from build123d import *

# Parameters (mm, degrees)
SKETCH1_R           = 3
BOSS_EXTRUDE2_DEPTH = 12.5
CUT_EXTRUDE1_DEPTH  = 2
SKETCH4_R           = 1.5
CUT_EXTRUDE4_DEPTH  = 2.5
SKETCH5_W           = 2.5
SKETCH5_H           = 4.5
BOSS_EXTRUDE3_DEPTH = 25
SKETCH6_R           = 1.500002847
CUT_EXTRUDE5_DEPTH  = 2.5
SKETCH7_R           = 1.1
CUT_EXTRUDE6_DEPTH  = 2


with BuildPart() as part:
    # Sketch1 → Boss-Extrude2 (new, symmetric)
    with BuildSketch(Plane.XY):
        Circle(SKETCH1_R)
        with BuildLine():
            Line((0, -3), (0, -0.5))
            Line((0, -0.5), (-17, -0.5))
            ThreePointArc((-17, -0.5), (-17.707106781, -0.792893219), (-18, -1.5))
            Line((-18, -1.5), (-18, -2))
            ThreePointArc((-18, -2), (-17.707106781, -2.707106781), (-17, -3))
            Line((-17, -3), (0, -3))
        make_face()
        Polygon((6.675258535, 32.098501889), (0.984807753, -0.173648178), (-0.984807753, 0.173648178), (4.705643029, 32.445798244), align=None)
    extrude(amount=BOSS_EXTRUDE2_DEPTH, both=True)

    # Sketch2 → Cut-Extrude1 (cut)
    with BuildSketch(Plane(origin=(0.9848077530122124, -0.17364817766692678, 0), x_dir=(0, 0, -1), z_dir=(0.9848077530122088, -0.17364817766692617, 0))):
        with BuildLine():
            Line((-8.6, 4.328427125), (8.6, 4.328427125))
            ThreePointArc((8.6, 4.328427125), (8.882842712, 4.445584412), (9, 4.728427125))
            Line((9, 4.728427125), (9, 4.928427125))
            ThreePointArc((9, 4.928427125), (8.882842712, 5.211269837), (8.6, 5.328427125))
            Line((8.6, 5.328427125), (-8.6, 5.328427125))
            ThreePointArc((-8.6, 5.328427125), (-8.882842712, 5.211269837), (-9, 4.928427125))
            Line((-9, 4.928427125), (-9, 4.728427125))
            ThreePointArc((-9, 4.728427125), (-8.882842712, 4.445584412), (-8.6, 4.328427125))
        make_face()
    extrude(amount=-CUT_EXTRUDE1_DEPTH, mode=Mode.SUBTRACT)

    # Sketch4 → Cut-Extrude4 (cut)
    with BuildSketch(Plane.XZ.offset(3)):
        with Locations((-6.562669804, 6.5)):
            Circle(SKETCH4_R)
        with Locations((-6.562669804, -6.5)):
            Circle(SKETCH4_R)
    extrude(amount=-CUT_EXTRUDE4_DEPTH, mode=Mode.SUBTRACT)

    # Sketch5 → Boss-Extrude3 (add)
    with BuildSketch(Plane.XY.offset(12.5)):
        with Locations((-1.25, -5.25)):
            Rectangle(SKETCH5_W, SKETCH5_H)
    extrude(amount=-BOSS_EXTRUDE3_DEPTH)

    # Sketch6 → Cut-Extrude5 (cut)
    with BuildSketch(Plane(origin=(0, 0, 0), x_dir=(0, 0, -1), z_dir=(1, 0, 0))):
        with Locations(Location((-8.822806399, -5.193294881, 0), (0, 0, 90))):
            Circle(SKETCH6_R)
    extrude(amount=-CUT_EXTRUDE5_DEPTH, mode=Mode.SUBTRACT)

    # Sketch7 → Cut-Extrude6 (cut)
    with BuildSketch(Plane(origin=(0.9848077530122124, -0.17364817766692678, 0), x_dir=(0, 0, -1), z_dir=(0.9848077530122088, -0.17364817766692617, 0))):
        with Locations(Location((-10.25, 30.52, 0), (0, 0, 90))):
            Circle(SKETCH7_R)
        with Locations(Location((-10.25, 17.02, 0), (0, 0, 90))):
            Circle(SKETCH7_R)
        with Locations(Location((10.25, 17.02, 0), (0, 0, 90))):
            Circle(SKETCH7_R)
        with Locations(Location((10.25, 30.52, 0), (0, 0, 90))):
            Circle(SKETCH7_R)
    extrude(amount=-CUT_EXTRUDE6_DEPTH, mode=Mode.SUBTRACT)


solid = part.part
Verification items for the finished model (mm, model axes). A direction names the side the tool comes from. Round coordinates to 2 decimals unless told otherwise and drop trailing zeros. Order: outer loops, then holes, each group sorted by start corner. A loop starts at its lowest first (then second) coordinate and runs counter-clockwise, first axis right, second up.
1. Section check B-B on z = -6.5. Record the cut outline in (x, y), then the cut area to 3 significant figures.
Final values:
outline: (-18, -2) arc R1 ccw to (-17, -3) - (-8.06, -3) - (-8.06, -0.5) - (-17, -0.5) arc R1 ccw to (-18, -1.5) - close; (-5.06, -3) - (-2.5, -3) - (-2.5, -7.5) - (0, -7.5) - (0, -3) arc R3 ccw to (1.48, 2.61) - (1.74, 4.09) - (-0.23, 4.44) - (-0.49, 2.96) arc R3 ccw to (-2.96, -0.5) - (-5.06, -0.5) - close; (-0.06, 5.42) - (1.91, 5.07) - (6.68, 32.1) - (4.71, 32.45) - close
area: 129 mm2
2. Thickness scan on L1, parallel to Y at x = -10.75, z = -9.5; L2, parallel to X at y = -5, z = -7; L3, parallel to X at y = 28, z = 6.5. Record the ranges inside material, lowest first.
Final values:
L1: y = -3 to -0.5
L2: x = -2.5 to 0
L3: x = 3.92 to 5.95
3. Section check D-D on x = -1. Record the cut outline in (y, z), then the cut area to 3 significant figures.
Final values:
outline: (-7.5, -12.5) - (2.83, -12.5) - (2.83, 12.5) - (-7.5, 12.5) - close; hole circle Ø3 at (-5.19, 8.82)
area: 251 mm2
4. Access from +Z, -Z, +X, -X, +Y, -Y to the whole of each face (thin tool, end or side, straight path). Record for faces 1 (the flat face through (-10, -3, 0)), 2 (the cylindrical face through (2.887, -0.816, 0.175)), 3 (the flat face through (0, -5, 0)), 4 (the flat face through (0.939, 5.245, -0.12)), 5 (the cylindrical face through (-1.23, -4.39, 10.09)).
Final values:
face 1: +Z, -Z, -X, -Y
face 2: +Z, -Z, +X
face 3: +Z, -Z, +X, -Y
face 4: -X
face 5: +X, -X
5. Go/stop test with flat-tipped pins: P1, Ø2, axis at x = 2.5, y = 26.5, coming from the +Z side; P2, Ø4, axis at y = 10, z = -4, coming from the -X side; P3, Ø4.5, axis at x = -11, z = 3, coming from the -Y side; P4, Ø6, axis at x = -8.5, z = -9, coming from the +Y side. Record where each tip stops, or that it passes through.
Final values:
P1: passes through
P2: stops at x = 0.4
P3: stops at y = -3
P4: stops at y = -0.5
6. Section check A-A on z = 1. Record the cut outline in (x, y).
Final values:
outline: (-18, -2) arc R1 ccw to (-17, -3) - (-2.5, -3) - (-2.5, -7.5) - (0, -7.5) - (0, -3) arc R3 ccw to (1.48, 2.61) - (1.74, 4.09) - (-0.23, 4.44) - (-0.49, 2.96) arc R3 ccw to (-2.96, -0.5) - (-17, -0.5) arc R1 ccw to (-18, -1.5) - close; (-0.06, 5.42) - (1.91, 5.07) - (6.68, 32.1) - (4.71, 32.45) - close
7. Section check C-C on x = -5.5. Record the cut outline in (y, z), then the cut area to 3 significant figures.
Final values:
outline: (-3, -12.5) - (-0.5, -12.5) - (-0.5, -7.56) - (-3, -7.56) - close; (-3, -5.44) - (-0.5, -5.44) - (-0.5, 5.44) - (-3, 5.44) - close; (-3, 7.56) - (-0.5, 7.56) - (-0.5, 12.5) - (-3, 12.5) - close
area: 51.9 mm2
8. Release check for a two-part mould opening along Y. For faces 6 (the cylindrical face through (-17.699, -0.785, 0.175)), 7 (the cylindrical face through (2.82, 15.9, 9.58)), 8 (the flat face through (1, 7, 12.5)) record: +Y half, -Y half, draft (parallel to the pull), parting line (faces both ways), or undercut.
Final values:
face 6: +Y half
face 7: undercut
face 8: draft
